Geometry: final body of the model. Coordinates: model frame, mm. A direction names the side the tool comes from. Give positions to 0.01 mm unless a question says otherwise; leave off trailing zeros. Order: outer loops, then holes, each group sorted by start corner. A loop starts at its lowest first (then second) coordinate and runs counter-clockwise, first axis right, second up. Notation, with made-up numbers: M 84.25,-20.75 L 120.25,-20.75 A17 cw 120.25,-9.75 Z; hole C -36,27 d9. An arc over 180 degrees is marked long. Write item = value, one per line. Start each with the question number.
from build123d import *

# Parameters (mm, degrees)
BOSS_EXTRUDE1_DEPTH = 10
SHELL1_T            = -1
BOSS_EXTRUDE2_DEPTH = 10
BOSS_EXTRUDE3_DEPTH = 10
SHELL3_START        = -10
SHELL3_DEPTH        = 9


# Read off the part's stored shape, not the designer's step: Shell3
with BuildPart() as part:
    # Sketch2 → Boss-Extrude1 (new body)
    with BuildSketch(Plane.XY):
        with BuildLine():
            Line((-11.25, 7.5), (11.25, 7.5))
            ThreePointArc((11.25, 7.5), (15.643398282, -3.106601718), (26.25, -7.5))
            Line((26.25, -7.5), (11.25, -7.5))
            Line((11.25, -7.5), (-11.25, -7.5))
            ThreePointArc((-11.25, -7.5), (-18.75, 0), (-11.25, 7.5))
        make_face()
    extrude(amount=-BOSS_EXTRUDE1_DEPTH)

    # Shell1
    shell1_openings = [part.faces().sort_by_distance(p)[0] for p in [
        (-1.202754878, -0.422571934, -10),
    ]]
    offset(amount=SHELL1_T, openings=shell1_openings, kind=Kind.INTERSECTION)

    # Sketch3 → Boss-Extrude2 (add)
    with BuildSketch(Plane.XY):
        Polygon((13.259618943, -5.5), (-11.25, -5.5), (-11.25, -6.5), (-11.25, -7.5), (13.259618943, -7.5), (13.259618943, -6.56903326), align=None)
    extrude(amount=-BOSS_EXTRUDE2_DEPTH)

    # Sketch6 → Boss-Extrude3 (add)
    with BuildSketch(Plane(origin=(0, 0, -10), x_dir=(-1, 0, 0), z_dir=(0, 0, -1))):
        with BuildLine():
            Line((-26.25, 20), (-26.25, 32.5))
            ThreePointArc((-26.25, 32.5), (-14.982652264, 29.088521604), (-7.5, 20))
            ThreePointArc((-7.5, 20), (-0.017347736, 10.911478396), (11.25, 7.5))
            Line((11.25, 7.5), (-11.25, 7.5))
            ThreePointArc((-11.25, 7.5), (-21.012812095, 11.034625486), (-26.25, 20))
        make_face()
    extrude(amount=-BOSS_EXTRUDE3_DEPTH)

    # Shell3 outline → Shell3 (cut)
    with BuildSketch(Plane.XY.offset(SHELL3_START)):
        with BuildLine():
            ThreePointArc((10.25, 7.5), (10.258344649, 8.016680893), (10.283369893, 8.532822846))
            ThreePointArc((10.283369893, 8.532822846), (19.960539936, 11.472190194), (25.25, 20.092463547))
            Line((25.25, 20.092463547), (25.25, 31.474092655))
            ThreePointArc((25.25, 31.474092655), (15.124781026, 27.973638192), (8.423076923, 19.615384615))
            ThreePointArc((8.423076923, 19.615384615), (3.148687527, 12.099433662), (-4.79825605, 7.5))
            Line((-4.79825605, 7.5), (10.25, 7.5))
        make_face()
    extrude(amount=SHELL3_DEPTH, mode=Mode.SUBTRACT)


solid = part.part
1) Pin query (flat end, axial travel): pin 1 Ø6 at (x, z) = (17, -6.5) entering from +Y; pin 2 Ø4 at (x, z) = (12.5, -1.5) entering from +Y; pin 3 Ø1.5 at (y, z) = (13, -2) entering from -X; pin 4 Ø12 at (x, y) = (12.5, 21) entering from -Z. Return the tip coordinate at first contact, or that it passes through.
2) Cut plane D-D (x = -9.5). Return loops of the section in (y, z).
3) Ray query, L1, parallel to Y at x = 15.5, z = -3; L2, parallel to Y at x = 10, z = -3 (1 decimal); L3, parallel to Y at x = 8.5, z = -6.75. Return the intervals inside material, ascending.
4) Cut plane C-C (y = 26.5). Return loops of the section in (x, z).
5) Draft query along Y for faces 1 (the flat face through (-1, 6.5, -5)), 2 (the flat face through (8, -7.5, -5)), 3 (the flat face through (26.25, 26, -5)). Return one class per face: pulls with the +Y half, pulls with the -Y half, needs draft (parallel to the pull), parting line crosses it, or undercut.
6) Access query for faces 4 (the flat face through (1, -5.5, -5)), 5 (the flat face through (7, 7, -10)), 6 (the cylindrical face through (15.53, -2.99, -4.93)). Directions: +Z, -Z, +X, -X, +Y, -Y. A direction counts if a zero-diameter tool reaches every point of the face in a straight line with its end or side. Return the directions, or none.
7) Cut plane A-A (z = -8). Give the number of separate pieces and of enclosed holes in the cut face, plus the area to 3 significant figures.
8) Cut plane B-B (x = 20.5). Return loops of the section in (y, z).
Reply:
q1.pin_1 = 31.51
q1.pin_2 = 28.76
q1.pin_3 = 1.8
q1.pin_4 = -10
q2.outline = M -7.5,-10 L -5.5,-10 L -5.5,-1 L 6.5,-1 L 6.5,-10 L 7.58,-10 L 7.58,0 L -7.5,0 Z
q3.L1 = -7.5 to -6.5, -4.35 to -2.96, 8.1 to 9.15, 28.23 to 29.42
q3.L2 = -7.5 to -5.5, 6.5 to 7.5, 22.6 to 24.4
q3.L3 = -7.5 to -5.5, 6.5 to 7.5, 19.8 to 22.06
q4.outline = M 11.84,-10 L 13.28,-10 L 13.28,-1 L 25.25,-1 L 25.25,-10 L 26.25,-10 L 26.25,0 L 11.84,0 Z
q5.face_1 = undercut
q5.face_2 = pulls with the -Y half
q5.face_3 = needs draft
q6.face_4 = -Z
q6.face_5 = -Z, +X, -X, +Y, -Y
q6.face_6 = +Z, -Z, +X
q7.separate_pieces = 1
q7.enclosed_holes = 2
q7.area = 196 mm²
q8.outline = M -7.5,-10 L -6.35,-10 L -6.35,0 L -7.5,0 Z; M 10.63,-10 L 11.91,-10 L 11.91,-1 L 30.62,-1 L 30.62,-10 L 31.67,-10 L 31.67,0 L 10.63,0 Z
